Check sheet for the modelled part. Datum: model origin and axes. Units: mm. Face numbers are marked on the shaded views. A direction names the side the tool comes from. Round coordinates to 2 decimals unless told otherwise and drop trailing zeros. Write each loop counter-clockwise with the first axis right and the second up, starting at its lowest first coordinate (ties: lowest second). Pieces come first, ordered by that corner, then holes. Notation, with made-up numbers: (-32.75, 8.25) - (13.25, 8.25) arc R26 cw to (13.25, 22.25) - close; hole circle Ø6 at (46.5, -13). An arc over 180 degrees is marked (long way). Use one line per item in the form item = value. Start each with the question number.
1) Gauge pin test, flat end, axial feed: P1, Ø8, axis at x = -30.5, y = -17.5, coming from the -Z side. Record the tip position at first contact, or that the pin passes through.
2) Section check A-A (z = -5). Record the boundary of the cut face in (x, y).
3) Set-up check for the marked faces 1 and 2: record each of +Z, -Z, +X, -X, +Y, -Y from which the full face is reachable in a straight line by a thin tool's end or side.
4) Section check C-C (x = -28). Record the boundary of the cut face in (y, z).
5) Scan lines: probe 1 along X at (y, z) = (-12, -4); probe 2 along Y at (x, z) = (-35, -2); probe 3 along Z at (x, y) = (-29, -15.5). Record each from-to range of solid material in increasing order.
6) Section check B-B (y = -8.5). Record the boundary of the cut face in (x, z), then the cut area to 4 significant figures.
7) Draft check along X on the marked faces 3, 4, 5 and 6. Enter one of: +X half, -X half, draft (parallel to the pull), parting line (faces both ways), or undercut.
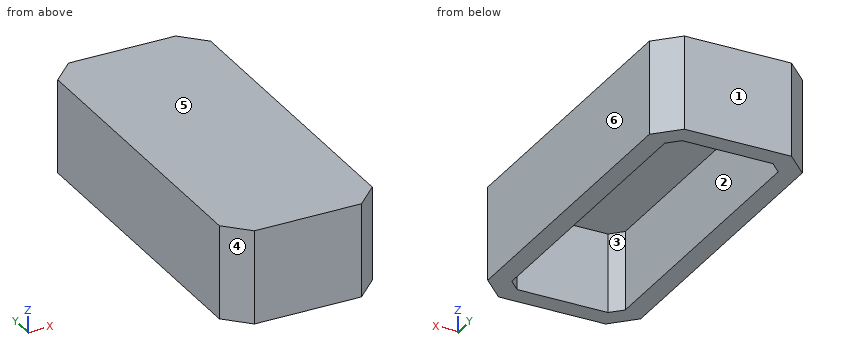
Autodesk Inventor part; units mm, degrees
ref_plane "YZ Plane" through (0, 0, 0) normal (1, 0, 0) x (0, 1, 0)
ref_plane "XZ Plane" through (0, 0, 0) normal (0, 1, 0) x (-1, 0, 0)
ref_plane "XY Plane" through (0, 0, 0) normal (0, 0, 1) x (1, 0, 0)
sketch "Sketch1" plane through (0, 0, 0) normal (0, 0, 1) x (1, 0, 0)
  line L0 (-35.5556, 1.5189) -> (-26.5556, 1.5189)
  line L1 (-25.5556, 0.5189) -> (-25.5556, -28.5811)
  line L2 (-26.5556, -29.5811) -> (-35.5556, -29.5811)
  line L3 (-36.5556, -28.5811) -> (-36.5556, 0.5189)
  line L4 (-35.5556, 1.5189) -> (-36.5556, 0.5189)
  line L5 (-25.5556, 0.5189) -> (-26.5556, 1.5189)
  line L6 (-25.5556, -28.5811) -> (-26.5556, -29.5811)
  line L7 (-35.5556, -29.5811) -> (-36.5556, -28.5811)
  line L8 (-26.452, 1.7689) -> (-25.3056, 0.6224)
  line L9 (-25.3056, 0.6224) -> (-25.3056, -28.6847)
  line L10 (-25.3056, -28.6847) -> (-26.452, -29.8311)
  line L11 (-26.452, -29.8311) -> (-35.6592, -29.8311)
  line L12 (-35.6592, -29.8311) -> (-36.8056, -28.6847)
  line L13 (-36.8056, -28.6847) -> (-36.8056, 0.6224)
  line L14 (-36.8056, 0.6224) -> (-35.6592, 1.7689)
  line L15 (-35.6592, 1.7689) -> (-26.452, 1.7689)
  line L16 (-25.6236, 3.7689) -> (-23.3056, 1.4508)
  line L17 (-23.3056, 1.4508) -> (-23.3056, -29.5131)
  line L18 (-23.3056, -29.5131) -> (-25.6236, -31.8311)
  line L19 (-25.6236, -31.8311) -> (-36.4876, -31.8311)
  line L20 (-36.4876, -31.8311) -> (-38.8056, -29.5131)
  line L21 (-38.8056, -29.5131) -> (-38.8056, 1.4508)
  line L22 (-38.8056, 1.4508) -> (-36.4876, 3.7689)
  line L23 (-36.4876, 3.7689) -> (-25.6236, 3.7689)
  point P0 (0, 0)
  point P1 (-36.5556, 1.5189)
  point P2 (-25.5556, -29.5811)
  point P3 (-25.5556, 1.5189)
  point P4 (-36.5556, -29.5811)
  dimension "d0" = 31.1
  dimension "d1" = 11
  dimension "d2" = 1
  dimension "d3" = 1
  dimension "d4" = 1
  dimension "d5" = 1
  dimension "d6" = 1
  dimension "d7" = 1
  dimension "d8" = 1
  dimension "d9" = 1
  dimension "d10" = 0.25
  dimension "d11" = 2
extrude "Extrusion1" add sketch "Sketch1" along normal blind 1.5 contours L0 L5 L1 L6 L2 L7 L3 L4 | L8 L9 L10 L11 L12 L13 L14 L15 | L16 L17 L18 L19 L20 L21 L22 L23
extrude "Extrusion2" add sketch "Sketch1" against normal blind 8 contours L16 L17 L18 L19 L20 L21 L22 L23
properties part number "CattailShellMockup_01"
Results are:
q1.P1 = 0
q2.outline = (-38.81, -29.51) - (-36.49, -31.83) - (-25.62, -31.83) - (-23.31, -29.51) - (-23.31, 1.45) - (-25.62, 3.77) - (-36.49, 3.77) - (-38.81, 1.45) - close; hole (-36.81, -28.68) - (-35.66, -29.83) - (-26.45, -29.83) - (-25.31, -28.68) - (-25.31, 0.62) - (-26.45, 1.77) - (-35.66, 1.77) - (-36.81, 0.62) - close
q3.face_1 = +Z, -Z, +X, -X, +Y
q3.face_2 = -Z
q4.outline = (-31.83, -8) - (-29.83, -8) - (-29.83, 0) - (1.77, 0) - (1.77, -8) - (3.77, -8) - (3.77, 1.5) - (-31.83, 1.5) - close
q5.probe_1 = -38.81 to -36.81, -25.31 to -23.31
q5.probe_2 = -31.83 to -29.83, 1.77 to 3.77
q5.probe_3 = 0 to 1.5
q6.outline = (-38.81, -8) - (-36.81, -8) - (-36.81, 0) - (-25.31, 0) - (-25.31, -8) - (-23.31, -8) - (-23.31, 1.5) - (-38.81, 1.5) - close
q6.area = 55.25 mm²
q7.face_3 = undercut
q7.face_4 = -X half
q7.face_5 = draft
q7.face_6 = +X half
